Here's the drawing with two shaded views (mm, measured from the low corner). I have some questions. Coordinates: 2 decimals unless noted, no trailing zeros. Write each loop counter-clockwise with the first axis right and the second up, starting at its lowest first coordinate (ties: lowest second). Pieces come first, ordered by that corner, then holes. Notation, with made-up numbers: (45.25, -34) -> (57.25, -34) arc R14 ccw to (57.25, -11) -> close; hole circle Ø11 at (67, 54.25). An arc over 180 degrees is marked (long way). Use a Markdown table: item, result. Add a question column.
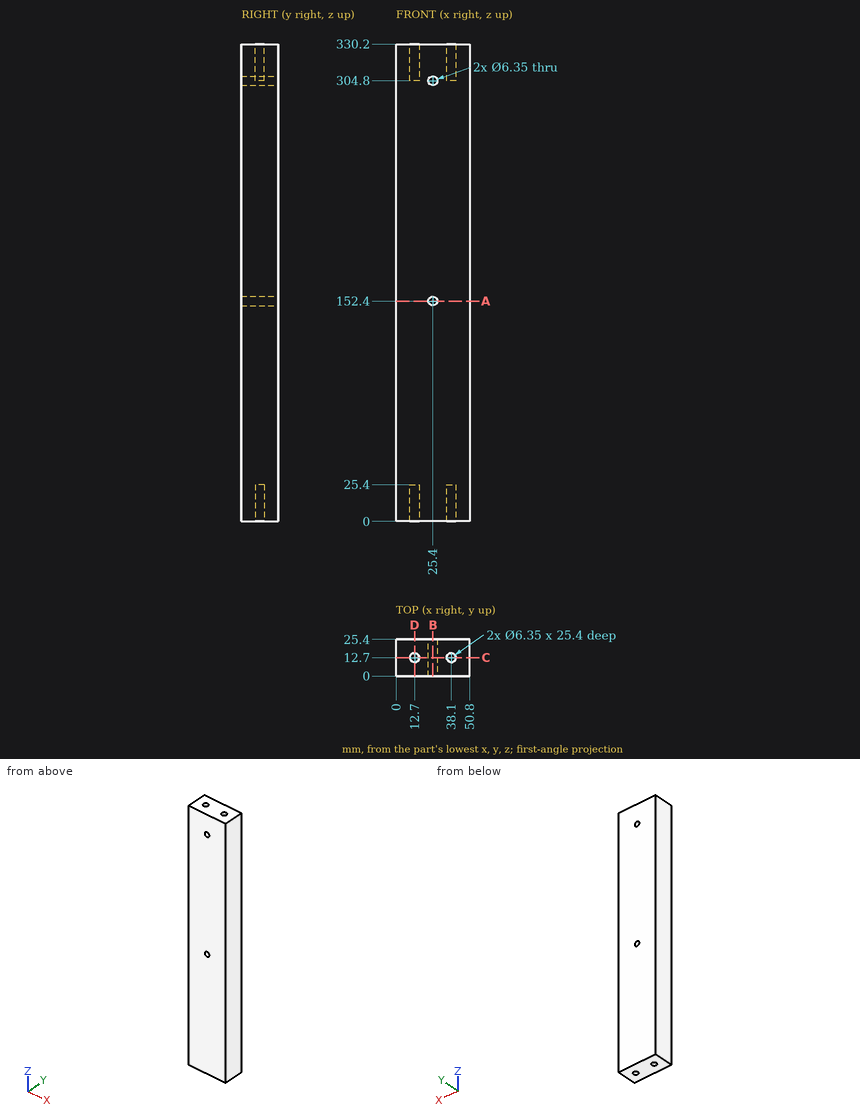
Q1. Suppose I cut it at C-C, the plane y = 12.7. Write out the boundary of the cut face in (x, z) (3 decimals), and give its area (3 significant figures).
Q2. Suppose I cut it at B-B, the plane x = 25.4. Write out the boundary of the cut face in (y, z) (3 decimals), and give its area (3 significant figures).
Q3. Suppose I cut it at D-D, the plane x = 12.7. Write out the boundary of the cut face in (y, z) (3 decimals), and give its area (3 significant figures).
Q4. Please list where these lines run through material, in increasing order: line 1 (Y direction, x = 38.1, z = 324) (3 decimals); line 2 (Z direction, x = 25.4, y = 16.75) (3 decimals); line 3 (Z direction, x = 24, y = 22).
Q5. Suppose I cut it at A-A, the plane z = 152.4. Write out the boundary of the cut face in (x, y) (3 decimals).
Q6. Will these pins go through, and if not, where does the flat tip stop? pin 1 (12 mm diameter, centred on x = 20, y = 5.5, fed in from -Z); pin 2 (1.9 mm diameter, centred on x = 36.5, y = 11.5, fed in from +Z).
Answer key:
| question | item | result |
|---|---|---|
| 1 | outline | (0, 0) -> (9.525, 0) -> (9.525, 25.4) -> (15.875, 25.4) -> (15.875, 0) -> (34.925, 0) -> (34.925, 25.4) -> (41.275, 25.4) -> (41.275, 0) -> (50.8, 0) -> (50.8, 330.2) -> (41.275, 330.2) -> (41.275, 304.8) -> (34.925, 304.8) -> (34.925, 330.2) -> (15.875, 330.2) -> (15.875, 304.8) -> (9.525, 304.8) -> (9.525, 330.2) -> (0, 330.2) -> close; hole circle Ø6.35 at (25.4, 152.4); hole circle Ø6.35 at (25.4, 304.8) |
| 1 | area | 16,100 mm^2 |
| 2 | outline | (0, 0) -> (25.4, 0) -> (25.4, 149.225) -> (0, 149.225) -> close; (0, 155.575) -> (25.4, 155.575) -> (25.4, 301.625) -> (0, 301.625) -> close; (0, 307.975) -> (25.4, 307.975) -> (25.4, 330.2) -> (0, 330.2) -> close |
| 2 | area | 8,060 mm^2 |
| 3 | outline | (0, 0) -> (9.525, 0) -> (9.525, 25.4) -> (15.875, 25.4) -> (15.875, 0) -> (25.4, 0) -> (25.4, 330.2) -> (15.875, 330.2) -> (15.875, 304.8) -> (9.525, 304.8) -> (9.525, 330.2) -> (0, 330.2) -> close |
| 3 | area | 8,060 mm^2 |
| 4 | line 1 | y = 0 to 9.525, 15.875 to 25.4 |
| 4 | line 2 | z = 0 to 149.225, 155.575 to 301.625, 307.975 to 330.2 |
| 4 | line 3 | z = 0 to 149.55, 155.25 to 301.95, 307.65 to 330.2 |
| 5 | outline | (0, 0) -> (22.225, 0) -> (22.225, 25.4) -> (0, 25.4) -> close; (28.575, 0) -> (50.8, 0) -> (50.8, 25.4) -> (28.575, 25.4) -> close |
| 6 | pin 1 | stops at z = 0 |
| 6 | pin 2 | stops at z = 304.8 |
